```python
from build123d import *

# Parameters (mm, degrees)
F1_DEPTH = 3.5
F2_W     = 1
F2_H     = 3.968627
F3_DEPTH = 25
F4_R     = 10
F5_DEPTH = 20
F6_R     = 2
F7_R     = 7.5
F8_DEPTH = 15


with BuildPart() as f1:
    # F0 (on Top) → F1 (new body)
    with BuildSketch(Plane.XY):
        Polygon((0, 2.5), (0, 0), (3.5, 0), (3.5, 2.5), (4, 2.5), (1.75, 4.484313), (-0.5, 2.5), align=None)
    extrude(amount=F1_DEPTH)

    # F2 (on face) → F3 (cut)
    with BuildSketch(Plane.XY.offset(3.5)):
        with Locations((1.75, 4.484313)):
            Rectangle(F2_W, F2_H)
        Polygon((1.25, 4.043355), (1.25, 2.5), (2.25, 2.5), (2.25, 4.043355), (1.75, 4.484313), align=None)
    extrude(amount=-F3_DEPTH, mode=Mode.SUBTRACT)

    # F4 (on face) → F5 (join)
    with BuildSketch(Plane.XZ):
        with Locations((1.75, 1.75)):
            Circle(F4_R)
    extrude(amount=F5_DEPTH)

    # F6
    f6_edges = [f1.edges().sort_by_distance(p)[0] for p in [
        (-8.25, 0, 1.75),
    ]]
    fillet(f6_edges, radius=F6_R)

    # F7 (on face) → F8 (cut)
    with BuildSketch(Plane.XZ.offset(20)):
        with Locations((1.75, 1.75)):
            Circle(F7_R)
    extrude(amount=-F8_DEPTH, mode=Mode.SUBTRACT)


solid = f1.part
```
Check sheet for the modelled part. Datum: model origin and axes. Units: mm. A direction names the side the tool comes from. Round coordinates to 2 decimals unless told otherwise and drop trailing zeros. Loops run counter-clockwise (first coordinate to the right, second up) from the corner with the lowest first, then second, coordinate; pieces in that order, holes last. Notation, with made-up numbers: (48.5, -18.75) -> (99.5, -18.75) arc R31 ccw to (99.5, 17.25) -> close; hole circle Ø2 at (65.5, 23). An arc over 180 degrees is marked (long way). Answer in a Markdown table with one row per item.
Q1. Go/stop test with flat-tipped pins: P1, Ø6, axis at x = 6, y = -14.5, coming from the -Z side; P2, Ø2, axis at x = 2.5, y = 1.5, coming from the +Z side; P3, Ø7.5, axis at x = 1, z = 3, coming from the -Y side. Record where each tip stops, or that it passes through.
Data:
| item | result |
|---|---|
| P1 | stops at z = -8.17 |
| P2 | stops at z = 3.5 |
| P3 | stops at y = -5 |
Q2. Thickness scan on L1, parallel to Z at x = 1.75, y = -7.75; L2, parallel to Z at x = 3.25, y = 2.25; L3, parallel to Z at x = -2.25, y = -18.5. Record the ranges inside material, lowest first.
Data:
| item | result |
|---|---|
| L1 | z = -8.25 to -5.75, 9.25 to 11.75 |
| L2 | z = 0 to 3.5 |
| L3 | z = -7.42 to -4.59, 8.09 to 10.92 |
Q3. Sectioned sample at A-A on x = 1.75. Enter the section's corners in (y, z), then the cut area to 3 significant figures.
Data:
| item | result |
|---|---|
| outline | (-20, -8.25) -> (-2, -8.25) arc R2 ccw to (0, -6.25) -> (0, 0) -> (2.5, 0) -> (2.5, 3.5) -> (0, 3.5) -> (0, 9.75) arc R2 ccw to (-2, 11.75) -> (-20, 11.75) -> (-20, 9.25) -> (-5, 9.25) -> (-5, -5.75) -> (-20, -5.75) -> close |
| area | 182 mm^2 |
Q4. Sectioned sample at B-B on y = 1.5. Enter the section's corners in (x, z), then the cut area to 4 significant figures.
Data:
| item | result |
|---|---|
| outline | (0, 0) -> (3.5, 0) -> (3.5, 3.5) -> (0, 3.5) -> close |
| area | 12.25 mm^2 |
Q5. Release check for a two-part mould opening along X. For faces 1 (the face through (2, 2.5, 2)), 2 (the face through (3.5, 1, 2)), 3 (the face through (5.4, -20, 8.5)) record: released by +X, released by -X, zero draft, split by the parting line, or undercut.
Data:
| item | result |
|---|---|
| face 1 | undercut |
| face 2 | released by +X |
| face 3 | zero draft |
Q6. Set-up check for faces 4 (the face through (-4.202, -12.605, -2.814)), 5 (the face through (2, 2, 0)), 6 (the face through (1.25, 3, 2)): record each of +Z, -Z, +X, -X, +Y, -Y from which the full face is reachable in a straight line by a thin tool's end or side.
Data:
| item | result |
|---|---|
| face 4 | -Y |
| face 5 | -Z, +X, -X, +Y |
| face 6 | +Z, -Z, +Y |
